from build123d import *

# Parameters (mm, degrees)
SKETCH1_R           = 14
BOSS_EXTRUDE1_DEPTH = 160
SKETCH2_R           = 10
BOSS_EXTRUDE2_DEPTH = 20


# Read off the part's stored shape, not the designer's step: M12x1.5 Machine Threads Stud1
with BuildPart() as part:
    # Sketch1 → Boss-Extrude1 (new body)
    with BuildSketch(Plane(origin=(0, 0, 0), x_dir=(1, 0, 0), z_dir=(0, 1, 0))):
        with Locations(Location((0, 0, 0), (0, 0, 270))):
            Circle(SKETCH1_R)
    extrude(amount=BOSS_EXTRUDE1_DEPTH)

    # Sketch2 → Boss-Extrude2 (add)
    with BuildSketch(Plane.XZ):
        with Locations(Location((0, 0, 0), (0, 0, 270))):
            Circle(SKETCH2_R)
    extrude(amount=BOSS_EXTRUDE2_DEPTH)

    # M12x1.5 Machine Threads Stud1 outline → M12x1.5 Machine Threads Stud1 (revolve, cut)
    with BuildSketch(Plane.XY):
        Polygon((10, 0), (6, 0), (6, -19.172), (5.172, -20), (10, -20), align=None)
    revolve(axis=Axis((0, 0, 0), (0, 1, 0)), mode=Mode.SUBTRACT)


solid = part.part
Build history of the part. All positions in model axes, mm. A direction names the side the tool comes from. Coordinates: 2 decimals unless noted, no trailing zeros. Write each loop counter-clockwise with the first axis right and the second up, starting at its lowest first coordinate (ties: lowest second). Pieces come first, ordered by that corner, then holes.
(1) Cut at D-D on x = -9.75. List the corners of the cut face in (y, z).
(2) 3-axis set-ups, long thin cutter, end or side, ignore diameter. For faces 1 (the cylindrical face through (-6, -10, 0)), 2 (the flat face through (0, -20, 0)): which of +Z, -Z, +X, -X, +Y, -Y reach the whole face in a straight line?
(3) Cut at B-B on z = 0. List the corners of the cut face in (x, y).
(4) Cut at A-A on x = 0. List the corners of the cut face in (y, z), and give its area (3 significant figures).
(5) Drill centre lines: line 1 (Y direction, x = -0.5, z = -7); line 2 (Z direction, x = 0.75, y = 87.5); line 3 (Z direction, x = -3, y = -7.5). Where is each one in solid material? Low to high.
(6) Cut at C-C on y = 42.5. List the corners of the cut face in (x, z).
(7) Pin check, flat tips, straight feed: pin 1 Ø2 at (y, z) = (80.5, -2.5) entering from -X; pin 2 Ø2 at (x, y) = (-11, 120.5) entering from -Z; pin 3 Ø8 at (y, z) = (110.5, -10) entering from +X. Stop position of each tip, or through.
Working result:
1. outline: (0, -10.05) - (160, -10.05) - (160, 10.05) - (0, 10.05) - close
2. face 1: -Y
2. face 2: +Z, -Z, +X, -X, -Y
3. outline: (-14, 0) - (-6, 0) - (-6, -19.17) - (-5.17, -20) - (5.17, -20) - (6, -19.17) - (6, 0) - (14, 0) - (14, 160) - (-14, 160) - close
4. outline: (-20, -5.17) - (-19.17, -6) - (0, -6) - (0, -14) - (160, -14) - (160, 14) - (0, 14) - (0, 6) - (-19.17, 6) - (-20, 5.17) - close
4. area: 4,720 mm2
5. line 1: y = 0 to 160
5. line 2: z = -13.98 to 13.98
5. line 3: z = -5.2 to 5.2
6. outline: circle Ø28 at (0, 0)
7. pin 1: stops at x = -13.92
7. pin 2: stops at z = -9.8
7. pin 3: stops at x = 12.65
